Here's the drawing with two shaded views (mm, measured from the low corner). I have some questions. A direction names the side the tool comes from. Coordinates: 2 decimals unless noted, no trailing zeros. Write each loop counter-clockwise with the first axis right and the second up, starting at its lowest first coordinate (ties: lowest second). Pieces come first, ordered by that corner, then holes.
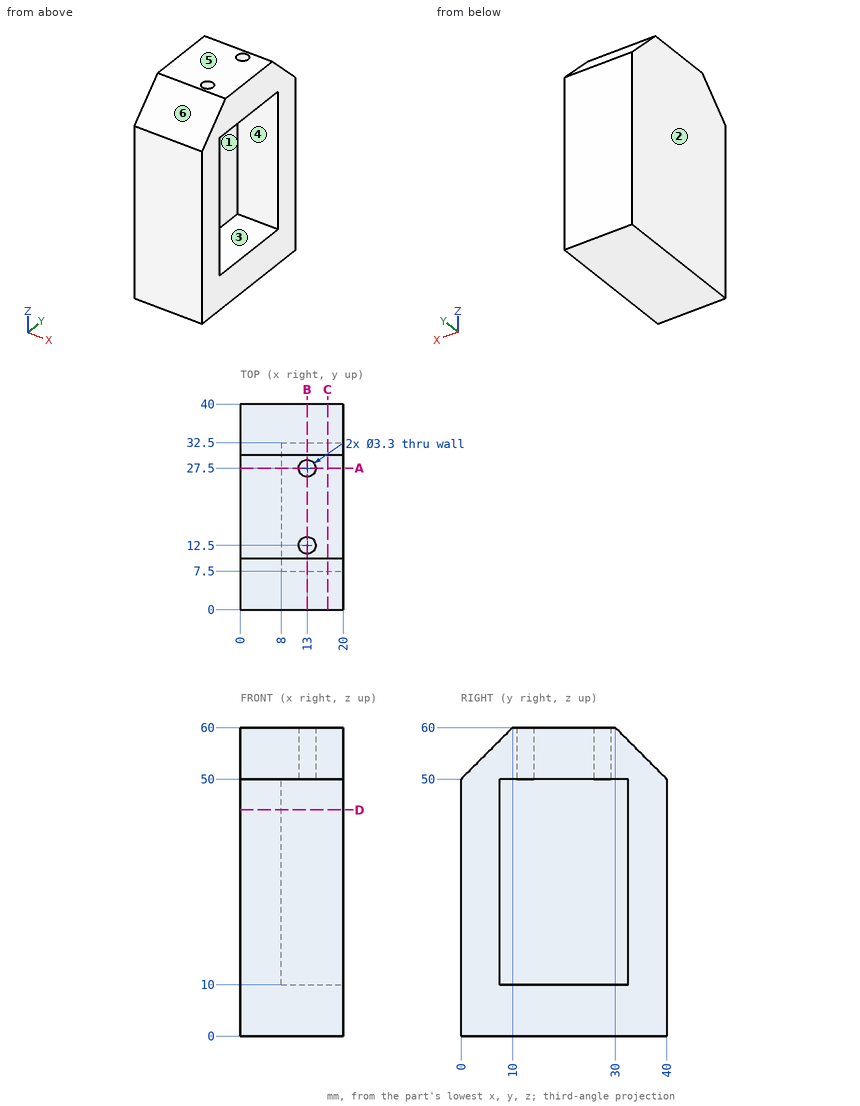
1. I want a section at A-A on y = 27.5. Please give me the cut outline in (x, z), plus the area to 3 significant figures.
Verdict:
outline: (0, 0) - (20, 0) - (20, 10) - (8, 10) - (8, 50) - (11.35, 50) - (11.35, 60) - (0, 60) - close; (14.65, 50) - (20, 50) - (20, 60) - (14.65, 60) - close
area: 687 mm2
2. On a 3-axis mill with a long thin cutter (end or side, diameter ignored), from which of +Z, -Z, +X, -X, +Y, -Y can I reach the whole of each face in a straight line? I mean the marked faces 1 and 2. Say none if no direction works.
Verdict:
face 1: +X
face 2: +Z, -Z, -X, +Y, -Y
3. I want a section at D-D on z = 44. Please give me the cut outline in (x, y).
Verdict:
outline: (0, 0) - (20, 0) - (20, 7.5) - (8, 7.5) - (8, 32.5) - (20, 32.5) - (20, 40) - (0, 40) - close
4. I want a section at C-C on x = 17. Please give me the cut outline in (y, z).
Verdict:
outline: (0, 0) - (40, 0) - (40, 50) - (30, 60) - (10, 60) - (0, 50) - close; hole (7.5, 10) - (32.5, 10) - (32.5, 50) - (7.5, 50) - close
5. If we mould it in two halves opening along Y, with no side actions, what happens to the marked faces 3, 4, 5 and 6? For each: pulls with the +Y half, pulls with the -Y half, needs draft (parallel to the pull), parting line crosses it, or undercut.
Verdict:
face 3: undercut
face 4: undercut
face 5: needs draft
face 6: pulls with the -Y half
6. I want a section at B-B on x = 13. Please give me the cut outline in (y, z), plus the area to 3 significant figures.
Verdict:
outline: (0, 0) - (40, 0) - (40, 50) - (30, 60) - (29.15, 60) - (29.15, 50) - (32.5, 50) - (32.5, 10) - (7.5, 10) - (7.5, 50) - (10.85, 50) - (10.85, 60) - (10, 60) - (0, 50) - close; (14.15, 50) - (25.85, 50) - (25.85, 60) - (14.15, 60) - close
area: 1,230 mm2
7. For pin 1 (10 mm diameter, centred on x = 13.5, z = 39.5, fed in from -Y); pin 2 (1 mm diameter, centred on y = 16, z = 29, fed in from +X); pin 3 (3 mm diameter, centred on x = 13, y = 12.5, fed in from +Z), each with a flat end and sliding along its axis, tell me the tip position at first contact or that it passes through.
Verdict:
pin 1: stops at y = 0
pin 2: stops at x = 8
pin 3: stops at z = 10
8. Please list where these lines run through material, in increasing order: line 1 along X through (y, z) = (12.5, 57); line 2 along Y through (x, z) = (8.5, 30.5); line 3 along Z through (x, y) = (10.75, 17.5).
Verdict:
line 1: x = 0 to 11.35, 14.65 to 20
line 2: y = 0 to 7.5, 32.5 to 40
line 3: z = 0 to 10, 50 to 60
